Build history of the part. All positions in model axes, mm. Face numbers are marked on the shaded views. Give positions to 0.01 mm unless a question says otherwise; leave off trailing zeros. Loops run counter-clockwise (first coordinate to the right, second up) from the corner with the lowest first, then second, coordinate; pieces in that order, holes last. Notation, with made-up numbers: (50.5, 43) - (99.5, 43) arc R31 ccw to (99.5, 82) - close; hole circle Ø9 at (53, 16). An arc over 180 degrees is marked (long way). Return JSON: item names as keys, results as strings. Group by question number.
1) Slice it at D-D (z = 18). List the corners of the cut face in (x, y), and give its area (3 significant figures).
2) Mould opens along Z. For the marked faces 1 and 2 say: released by +Z, released by -Z, zero draft, split by the parting line, or undercut.
3) Drop flat-ended pins along their axis: pin 1 (0.6 mm diameter, centred on x = 13.5, y = 0.5, fed in from -Z); pin 2 (1 mm diameter, centred on x = 5.5, y = 1.5, fed in from -Z); pin 3 (0.6 mm diameter, centred on y = 1, z = 11.5, fed in from -X). Give the stop position or say it passes through.
4) Slice it at A-A (x = 0). List the corners of the cut face in (y, z), and give its area (3 significant figures).
5) Drill centre lines: probe 1 along Z at (x, y) = (17, 0.7); probe 2 along Z at (x, y) = (-1.5, 0.5); probe 3 along X at (y, z) = (1.8, -14). Where is each one in solid material? Low to high. Write a range as from..to.
6) Slice it at C-C (y = 0.95). Count the separate pieces of the cut face and the enclosed holes in it, and give its area (3 significant figures).
7) Slice it at B-B (z = 0). List the corners of the cut face in (x, y).
```python
from build123d import *

# Parameters (mm, degrees)
SKETCH1_R                                      = 5
BOSS_EXTRUDE1_DEPTH                            = 2
M3_CLEARANCE_HOLE1_D                           = 3.4
CSK_FOR_M3_FLAT_HEAD_MACHINE_SCREW3_AT_2_COUNT = 2
CSK_FOR_M3_FLAT_HEAD_MACHINE_SCREW3_AT_2_PITCH = 12.419742348
CSK_FOR_M3_FLAT_HEAD_MACHINE_SCREW3_AT_3_COUNT = 2
CSK_FOR_M3_FLAT_HEAD_MACHINE_SCREW3_AT_3_PITCH = 16
CSK_FOR_M3_FLAT_HEAD_MACHINE_SCREW3_AT_4_COUNT = 2
CSK_FOR_M3_FLAT_HEAD_MACHINE_SCREW3_AT_4_PITCH = 12.419742348


with BuildPart() as part:
    # Sketch1 → Boss-Extrude1 (new body)
    with BuildSketch(Plane(origin=(0, 0, 0), x_dir=(1, 0, 0), z_dir=(0, 1, 0))):
        with BuildLine():
            Line((3.5, 9.5), (3.5, 17))
            ThreePointArc((3.5, 17), (0, 20.5), (-3.5, 17))
            Line((-3.5, 17), (-3.5, 9.5))
            ThreePointArc((-3.5, 9.5), (-5.257359313, 5.257359313), (-9.5, 3.5))
            Line((-9.5, 3.5), (-17, 3.5))
            ThreePointArc((-17, 3.5), (-20.5, 0), (-17, -3.5))
            Line((-17, -3.5), (-9.5, -3.5))
            ThreePointArc((-9.5, -3.5), (-5.257359313, -5.257359313), (-3.5, -9.5))
            Line((-3.5, -9.5), (-3.5, -17))
            ThreePointArc((-3.5, -17), (0, -20.5), (3.5, -17))
            Line((3.5, -17), (3.5, -9.5))
            ThreePointArc((3.5, -9.5), (5.257359313, -5.257359313), (9.5, -3.5))
            Line((9.5, -3.5), (17, -3.5))
            ThreePointArc((17, -3.5), (20.5, 0), (17, 3.5))
            Line((17, 3.5), (9.5, 3.5))
            ThreePointArc((9.5, 3.5), (5.257359313, 5.257359313), (3.5, 9.5))
        make_face()
        with Locations(Location((0, 0, 0), (0, 0, 270))):
            Circle(SKETCH1_R, mode=Mode.SUBTRACT)
    extrude(amount=BOSS_EXTRUDE1_DEPTH)

    # M3 Clearance Hole1 (through all)
    with Locations(Plane(origin=(0, 2, 0), x_dir=(1, 0, 0), z_dir=(0, 1, 0))):
        with Locations((0, 17), (-17, 0), (17, 0), (0, -17)):
            Hole(M3_CLEARANCE_HOLE1_D / 2)

    # Sketch8 → CSK for M3 Flat Head Machine Screw3 (revolve, cut)
    with BuildSketch(Plane(origin=(0, 2, -8), x_dir=(0, 0, 1), z_dir=(1, 0, 0))):
        Polygon((0, 0), (0, 2), (1.7, 2), (1.7, 1.45), (3.15, 0), align=None)
    csk_for_m3_flat_head_machine_screw3 = revolve(axis=Axis((0, 8.35, -8), (0, -1, 0)), mode=Mode.SUBTRACT)

    # CSK for M3 Flat Head Machine Screw3 at 2: CSK for M3 Flat Head Machine Screw3 ×2
    with Locations(*[Vector(-0.7649111981170509, 0, 0.6441357457827798) * (i * CSK_FOR_M3_FLAT_HEAD_MACHINE_SCREW3_AT_2_PITCH) for i in range(1, CSK_FOR_M3_FLAT_HEAD_MACHINE_SCREW3_AT_2_COUNT)]):
        add(csk_for_m3_flat_head_machine_screw3, mode=Mode.SUBTRACT)

    # CSK for M3 Flat Head Machine Screw3 at 3: CSK for M3 Flat Head Machine Screw3 ×2
    with Locations(*[(0, 0, i * CSK_FOR_M3_FLAT_HEAD_MACHINE_SCREW3_AT_3_PITCH) for i in range(1, CSK_FOR_M3_FLAT_HEAD_MACHINE_SCREW3_AT_3_COUNT)]):
        add(csk_for_m3_flat_head_machine_screw3, mode=Mode.SUBTRACT)

    # CSK for M3 Flat Head Machine Screw3 at 4: CSK for M3 Flat Head Machine Screw3 ×2
    with Locations(*[Vector(0.7649111981170508, 0, 0.6441357457827798) * (i * CSK_FOR_M3_FLAT_HEAD_MACHINE_SCREW3_AT_4_PITCH) for i in range(1, CSK_FOR_M3_FLAT_HEAD_MACHINE_SCREW3_AT_4_COUNT)]):
        add(csk_for_m3_flat_head_machine_screw3, mode=Mode.SUBTRACT)


solid = part.part
```
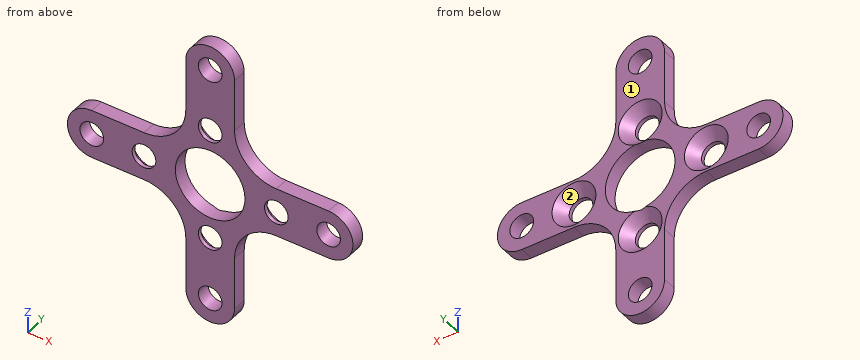
Results:
{
 "1": {"outline": "(-3.35, 0) - (-1.37, 0) - (-1.37, 2) - (-3.35, 2) - close; (1.37, 0) - (3.35, 0) - (3.35, 2) - (1.37, 2) - close", "area": "7.92 mm2"},
 "2": {"face 1": "zero draft", "face 2": "undercut"},
 "3": {"pin 1": "z = -3.5", "pin 2": "z = -5.53", "pin 3": "x = -3.5"},
 "4": {"outline": "(0, -20.5) - (2, -20.5) - (2, -18.7) - (0, -18.7) - close; (0, -15.3) - (2, -15.3) - (2, -11.15) - (0.55, -9.7) - (0, -9.7) - close; (0, -6.3) - (0.55, -6.3) - (1.85, -5) - (0, -5) - close; (0, 5) - (1.85, 5) - (0.55, 6.3) - (0, 6.3) - close; (0, 9.7) - (0.55, 9.7) - (2, 11.15) - (2, 15.3) - (0, 15.3) - close; (0, 18.7) - (2, 18.7) - (2, 20.5) - (0, 20.5) - close", "area": "30.6 mm2"},
 "5": {"probe 1": "-3.5..-1.7, 1.7..3.5", "probe 2": "-20.16..-17.8, -16.2..-8.8, -7.2..-4.77, 4.77..7.2, 8.8..16.2, 17.8..20.16", "probe 3": "-3.5..3.5"},
 "6": {"separate pieces": "1", "enclosed holes": "9", "area": "365 mm2"},
 "7": {"outline": "(-20.5, 0) - (-18.7, 0) - (-18.7, 2) - (-20.5, 2) - close; (-15.3, 0) - (-11.2, 0) - (-11.2, 0.55) - (-12.65, 2) - (-15.3, 2) - close; (-7.8, 0) - (-5, 0) - (-5, 2) - (-6.35, 2) - (-7.8, 0.55) - close; (5, 0) - (7.8, 0) - (7.8, 0.55) - (6.35, 2) - (5, 2) - close; (11.2, 0) - (15.3, 0) - (15.3, 2) - (12.65, 2) - (11.2, 0.55) - close; (18.7, 0) - (20.5, 0) - (20.5, 2) - (18.7, 2) - close"}
}
